```python
from build123d import *

# Parameters (mm, degrees)
EXTRUDE_1_DEPTH     = 12
EXTRUDE_2_DEPTH     = 24
SKETCH_6_W          = 3
SKETCH_6_H          = 15
EXTRUDE_3_DEPTH     = 12
EXTRUDE_4_DEPTH     = 24
CUT_EXTRUDE_4_DEPTH = 267.326866838
CUT_EXTRUDE_5_DEPTH = 265.954713112
FILLET_1_R          = 2


with BuildPart() as part:
    # 草图1 → 凸台-拉伸1 (new body)
    with BuildSketch(Plane(origin=(0, 0, 0), x_dir=(1, 0, 0), z_dir=(0, 1, 0))):
        Polygon((-123, 2), (-123, 0), (0, 0), (0, 24), (-123, 24), (-123, 22), (-113.5, 22), (-113.5, 20), (-110.5, 20), (-110.5, 22), (-90, 22), (-90, 2), (-110.5, 2), (-110.5, 4), (-113.5, 4), (-113.5, 2), align=None)
    extrude(amount=EXTRUDE_1_DEPTH)

    # 草图5 → 凸台-拉伸2 (add)
    with BuildSketch(Plane(origin=(0, 0, -24), x_dir=(-1, 0, 0), z_dir=(0, 0, -1))):
        with BuildLine():
            Line((0, 0), (12, 0))
            Line((12, 0), (12, 183))
            ThreePointArc((12, 183), (23.715728753, 211.284271247), (52, 223))
            Line((52, 223), (120, 223))
            Line((120, 223), (120, 235))
            Line((120, 235), (40, 235))
            ThreePointArc((40, 235), (11.715728753, 223.284271247), (0, 195))
            Line((0, 195), (0, 0))
        make_face()
    extrude(amount=-EXTRUDE_2_DEPTH)

    # 草图6 → 凸台-拉伸3 (add)
    with BuildSketch(Plane.XZ.offset(-223)):
        with Locations((-107.5, -12)):
            Rectangle(SKETCH_6_W, SKETCH_6_H)
        with Locations((-92.5, -12)):
            Rectangle(SKETCH_6_W, SKETCH_6_H)
    extrude(amount=EXTRUDE_3_DEPTH)

    # 草图7 → 凸台-拉伸4 (add)
    with BuildSketch(Plane(origin=(0, 0, -24), x_dir=(-1, 0, 0), z_dir=(0, 0, -1))):
        with BuildLine():
            Line((32, 12), (12, 12))
            Line((12, 12), (12, 32))
            ThreePointArc((12, 32), (17.857864376, 17.857864376), (32, 12))
        make_face()
    extrude(amount=-EXTRUDE_4_DEPTH)

    # 草图8 → 切除-拉伸4 (cut, through all)
    with BuildSketch(Plane(origin=(0, 0, -24), x_dir=(-1, 0, 0), z_dir=(0, 0, -1))):
        with BuildLine():
            Line((0, 20), (0, 0))
            Line((0, 0), (20, 0))
            ThreePointArc((20, 0), (5.857864376, 5.857864376), (0, 20))
        make_face()
    extrude(amount=-CUT_EXTRUDE_4_DEPTH, mode=Mode.SUBTRACT)

    # 草图9 → 切除-拉伸5 (cut, through all)
    with BuildSketch(Plane.ZY.offset(120)):
        with BuildLine():
            Line((-24, 235), (-24, 223))
            ThreePointArc((-24, 223), (-23.182219831, 229.211657082), (-20.784609691, 235))
            Line((-20.784609691, 235), (-24, 235))
        make_face()
    extrude(amount=-CUT_EXTRUDE_5_DEPTH, mode=Mode.SUBTRACT)

    # 圆角1
    fillet_1_edges = [part.edges().sort_by_distance(p)[0] for p in [
        (-109, 211, -12),
        (-91, 211, -12),
    ]]
    fillet(fillet_1_edges, radius=FILLET_1_R)


solid = part.part
```
Work out the finished part from the listing and answer in its coordinate system (mm). A direction names the side the tool comes from. Give positions to 0.01 mm unless a question says otherwise; leave off trailing zeros. Write each loop counter-clockwise with the first axis right and the second up, starting at its lowest first coordinate (ties: lowest second). Pieces come first, ordered by that corner, then holes. Notation, with made-up numbers: (51, 11) -> (64, 11) arc R15 ccw to (64, 23) -> close; hole circle Ø8 at (-11, 84.25). An arc over 180 degrees is marked (long way). Write item = value, one per line.
Q1. Section C-C on y = 216 is taken. Determine the outline of the cut face in (x, z).
Computed values:
outline = (-109, -19.5) -> (-106, -19.5) -> (-106, -4.5) -> (-109, -4.5) -> close; (-94, -19.5) -> (-91, -19.5) -> (-91, -4.5) -> (-94, -4.5) -> close; (-29.39, -24) -> (-5.96, -24) -> (-5.96, 0) -> (-29.39, 0) -> close
Q2. Section B-B on z = -17 is taken. Determine the outline of the cut face in (x, y), and give its area (3 significant figures).
Computed values:
outline = (-120, 223) -> (-109, 223) -> (-109, 213) arc R2 ccw to (-107, 211) -> (-106, 211) -> (-106, 223) -> (-94, 223) -> (-94, 211) -> (-93, 211) arc R2 ccw to (-91, 213) -> (-91, 223) -> (-52, 223) arc R40 cw to (-12, 183) -> (-12, 32) arc R20 cw to (-32, 12) -> (-90, 12) -> (-90, 0) -> (-20, 0) arc R20 ccw to (0, 20) -> (0, 195) arc R40 ccw to (-40, 235) -> (-120, 235) -> close
area = 5,120 mm^2
Q3. A tool of negligible diameter and unlimited length cuts with its end or side. For faces 1 (the flat face through (-100, 6, -2)), 2 (the cylindrical face through (-23.406, 210.972, -12.168)), 3 (the flat face through (-106, 217, -12)), from which of +Z, -Z, +X, -X, +Y, -Y can it reach the whole face along a straight path? Write none if from no direction.
Computed values:
face_1 = -Y
face_2 = +Z, -Z
face_3 = +Z, -Z, -Y
Q4. For a pull along Z with two mould halves and no side action, classify faces 4 (the flat face through (-11.7, 126.8, 0)), 5 (the cylindrical face through (-17.703, 18.014, -12.168)), 6 (the flat face through (-100, 6, -22)) as pulls with the +Z half, pulls with the -Z half, needs draft (parallel to the pull), parting line crosses it, or undercut.
Computed values:
face_4 = pulls with the +Z half
face_5 = needs draft
face_6 = undercut
Q5. Section A-A on x = -54.5 is taken. Determine the outline of the cut face in (y, z).
Computed values:
outline = (0, -24) -> (12, -24) -> (12, 0) -> (0, 0) -> close; (223, -24) arc R24 ccw to (235, -20.78) -> (235, 0) -> (223, 0) -> close
Q6. Flat-ended cylindrical pins translate along their axes: pin 1 Ø13 at (y, z) = (230.5, -11.5) entering from -X; pin 2 Ø0.8 at (x, z) = (-106.5, -12) entering from -Y; pin 3 Ø1.5 at (x, y) = (-108, 216.5) entering from +Z. Find the tip coordinate at first contact, or state that the pin passes through.
Computed values:
pin_1 = -120
pin_2 = 211
pin_3 = -4.5
Q7. Consider line 1 along Y through (x, z) = (-54.5, -20); line 2 along X through (y, z) = (217.5, -6); line 3 along Y through (x, z) = (-98.5, -12.5). Determine where each line is inside the solid, lowest interval first.
Computed values:
line_1 = 0 to 12, 223 to 235
line_2 = -109 to -106, -94 to -91, -31.76 to -6.93
line_3 = 223 to 235
Q8. Section D-D on y = 114.5 is taken. Determine the outline of the cut face in (x, z).
Computed values:
outline = (-12, -24) -> (0, -24) -> (0, 0) -> (-12, 0) -> close
